Source: three-view drawing plus pictorial views. Frame: mm from the lowest corner of the part. A direction names the side the tool comes from. Give positions to 0.01 mm unless a question says otherwise; leave off trailing zeros. Write each loop counter-clockwise with the first axis right and the second up, starting at its lowest first coordinate (ties: lowest second). Pieces come first, ordered by that corner, then holes. Notation, with made-up numbers: (-21.75, -2.5) -> (-5.75, -2.5) arc R23 cw to (-5.75, 21.5) -> close; hole circle Ø8 at (49.25, 72.5). An arc over 180 degrees is marked (long way). Write item = value, one per line.
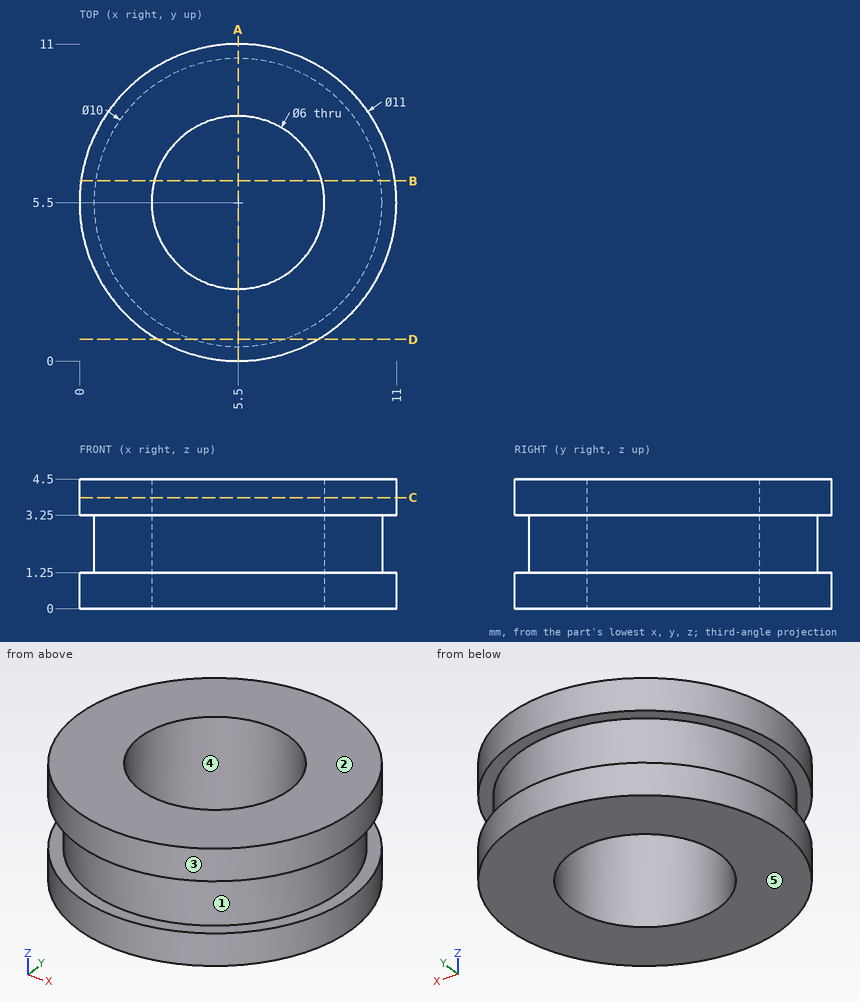
1) Material intervals for L1, parallel to Z at x = 7.25, y = 10.5; L2, parallel to Y at x = 5.5, z = 3.65; L3, parallel to X at y = 2.75, z = 3.2, sorted ascending.
Computed:
L1 = 0 to 1.25, 3.25 to 4.5
L2 = 0 to 2.5, 8.5 to 11
L3 = 1.32 to 4.3, 6.7 to 9.68
2) Access query for the marked faces 1 and 2. Directions: +Z, -Z, +X, -X, +Y, -Y. A direction counts if a zero-diameter tool reaches every point of the face in a straight line with its end or side. Return the directions, or none.
Computed:
face_1 = none
face_2 = +Z, +X, -X, +Y, -Y
3) Cut plane B-B (y = 6.25). Return the cut outline in (x, z), then the cut area to 3 significant figures.
Computed:
outline = (0.05, 0) -> (2.6, 0) -> (2.6, 4.5) -> (0.05, 4.5) -> (0.05, 3.25) -> (0.56, 3.25) -> (0.56, 1.25) -> (0.05, 1.25) -> close; (8.4, 0) -> (10.95, 0) -> (10.95, 1.25) -> (10.44, 1.25) -> (10.44, 3.25) -> (10.95, 3.25) -> (10.95, 4.5) -> (8.4, 4.5) -> close
area = 20.9 mm²
4) Cut plane D-D (y = 0.75). Return the cut outline in (x, z).
Computed:
outline = (2.73, 0) -> (8.27, 0) -> (8.27, 1.25) -> (7.06, 1.25) -> (7.06, 3.25) -> (8.27, 3.25) -> (8.27, 4.5) -> (2.73, 4.5) -> (2.73, 3.25) -> (3.94, 3.25) -> (3.94, 1.25) -> (2.73, 1.25) -> close
5) Draft query along Y for the marked faces 3, 4 and 5. Return one class per face: pulls with the +Y half, pulls with the -Y half, needs draft (parallel to the pull), parting line crosses it, or undercut.
Computed:
face_3 = parting line crosses it
face_4 = undercut
face_5 = needs draft
6) Contact query for flat-ended pins moving along their axis: pin 1 (1.5 mm diameter, centred on y = 1, z = 1, fed in from +X); pin 2 (3.5 mm diameter, centred on x = 5.5, y = 5.5, fed in from -Z). Output: stop coordinate, or through.
Computed:
pin_1 = 9.52
pin_2 = through
7) Cut plane C-C (z = 3.85). Return the cut outline in (x, y), then the cut area to 3 significant figures.
Computed:
outline = circle Ø11 at (5.5, 5.5); hole circle Ø6 at (5.5, 5.5)
area = 66.8 mm²
8) Cut plane A-A (x = 5.5). Return the cut outline in (y, z), then the cut area to 3 significant figures.
Computed:
outline = (0, 0) -> (2.5, 0) -> (2.5, 4.5) -> (0, 4.5) -> (0, 3.25) -> (0.5, 3.25) -> (0.5, 1.25) -> (0, 1.25) -> close; (8.5, 0) -> (11, 0) -> (11, 1.25) -> (10.5, 1.25) -> (10.5, 3.25) -> (11, 3.25) -> (11, 4.5) -> (8.5, 4.5) -> close
area = 20.5 mm²
